Geometry check sheet. Reference: the model listing, model coordinates, mm. Face numbers are marked on the shaded views. A direction names the side the tool comes from. Round coordinates to 2 decimals unless told otherwise and drop trailing zeros. Loops run counter-clockwise (first coordinate to the right, second up) from the corner with the lowest first, then second, coordinate; pieces in that order, holes last.
```python
from build123d import *
from build123d.topology import SkipClean

# Parameters (mm, degrees)
ESQUISSE1_R        = 75
ESQUISSE1_R_2      = 2
BOSS_EXTRU_1_DEPTH = 10
ESQUISSE2_R        = 2
ESQUISSE2_W        = 21
ESQUISSE2_H        = 41
ESQUISSE2_H_2      = 6.85
BOSS_EXTRU_2_DEPTH = 2
BOSS_EXTRU_5_START = 2
ESQUISSE2_7_R      = 2
BOSS_EXTRU_5_DEPTH = 8


with BuildPart() as part:
    # Esquisse1 → Boss.-Extru.1 (new body)
    with BuildSketch(Plane(origin=(0, 0, 0), x_dir=(1, 0, 0), z_dir=(0, 1, 0))):
        with Locations(Location((0, 0, 0), (0, 0, 270))):
            Circle(ESQUISSE1_R)
        with Locations(Location((0, 65, 0), (0, 0, 270))):
            Circle(ESQUISSE1_R_2, mode=Mode.SUBTRACT)
        with Locations(Location((0, -65, 0), (0, 0, 270))):
            Circle(ESQUISSE1_R_2, mode=Mode.SUBTRACT)
    extrude(amount=BOSS_EXTRU_1_DEPTH)

    # Esquisse2 → Boss.-Extru.2 (add)
    # profile 1 of 3: a face of its own
    with BuildSketch(Plane.XY):
        with BuildLine():
            ThreePointArc((-25.073934757, 16.568086991), (-23.205708304, 20.950030541), (-23.576750129, 25.699138596))
            Line((-23.576750129, 25.699138596), (-28.491553882, 40.606845184))
            ThreePointArc((-28.491553882, 40.606845184), (0, 80), (28.491553882, 40.606845184))
            Line((28.491553882, 40.606845184), (23.576750129, 25.699138596))
            ThreePointArc((23.576750129, 25.699138596), (23.205708304, 20.950030541), (25.073934757, 16.568086991))
            Line((25.073934757, 16.568086991), (30, 10))
            Line((30, 10), (-30, 10))
            Line((-30, 10), (-25.073934757, 16.568086991))
        make_face()
        with Locations((4.751288604, 21.76470447)):
            Circle(ESQUISSE2_R, mode=Mode.SUBTRACT)
        with Locations((-5.248711396, 21.76470447)):
            Circle(ESQUISSE2_R, mode=Mode.SUBTRACT)
        with Locations((-5.248711396, 70.39470447)):
            Circle(ESQUISSE2_R, mode=Mode.SUBTRACT)
        with Locations((4.751288604, 70.39470447)):
            Circle(ESQUISSE2_R, mode=Mode.SUBTRACT)
        with Locations((-0.248711396, 46.01543183)):
            Rectangle(ESQUISSE2_W, ESQUISSE2_H, mode=Mode.SUBTRACT)
    # profile 2 of 3: a face of its own
    with BuildSketch(Plane.XY):
        with Locations((-0.248711396, 69.94043183)):
            Rectangle(ESQUISSE2_W, ESQUISSE2_H_2)
        with Locations((-5.248711396, 70.39470447)):
            Circle(ESQUISSE2_R, mode=Mode.SUBTRACT)
        with Locations((4.751288604, 70.39470447)):
            Circle(ESQUISSE2_R, mode=Mode.SUBTRACT)
    # profile 3 of 3: a face of its own
    with BuildSketch(Plane.XY):
        with BuildLine():
            Line((10.251288604, 73.36543183), (10.251288604, 78.194167517))
            ThreePointArc((10.251288604, 78.194167517), (-0.265506097, 79.998825086), (-10.748711396, 78.00830597))
            Line((-10.748711396, 78.00830597), (-10.748711396, 73.36543183))
            Line((-10.748711396, 73.36543183), (10.251288604, 73.36543183))
        make_face()
    extrude(amount=BOSS_EXTRU_2_DEPTH)

    # Esquisse2<7> → Boss.-Extru.5 (add)
    with SkipClean():  # the faces are left unmerged after this step: merging them gives an invalid solid
        with BuildSketch(Plane.XY.offset(BOSS_EXTRU_5_START)):
            with BuildLine():
                Line((23.576750129, 25.699138596), (28.491553882, 40.606845184))
                ThreePointArc((28.491553882, 40.606845184), (26.989880715, 63.097569965), (10.251288604, 78.194167517))
                Line((10.251288604, 78.194167517), (10.251288604, 73.36543183))
                Line((10.251288604, 73.36543183), (10.251288604, 66.51543183))
                Line((10.251288604, 66.51543183), (10.251288604, 25.51543183))
                Line((10.251288604, 25.51543183), (-10.748711396, 25.51543183))
                Line((-10.748711396, 25.51543183), (-10.748711396, 66.51543183))
                Line((-10.748711396, 66.51543183), (-10.748711396, 73.36543183))
                Line((-10.748711396, 73.36543183), (-10.748711396, 78.00830597))
                ThreePointArc((-10.748711396, 78.00830597), (-27.104739844, 62.858191085), (-28.491553882, 40.606845184))
                Line((-28.491553882, 40.606845184), (-23.576750129, 25.699138596))
                ThreePointArc((-23.576750129, 25.699138596), (-23.205708304, 20.950030541), (-25.073934757, 16.568086991))
                Line((-25.073934757, 16.568086991), (-30, 10))
                Line((-30, 10), (30, 10))
                Line((30, 10), (25.073934757, 16.568086991))
                ThreePointArc((25.073934757, 16.568086991), (23.205708304, 20.950030541), (23.576750129, 25.699138596))
            make_face()
            with Locations((-5.248711396, 21.76470447)):
                Circle(ESQUISSE2_7_R, mode=Mode.SUBTRACT)
            with Locations((4.751288604, 21.76470447)):
                Circle(ESQUISSE2_7_R, mode=Mode.SUBTRACT)
        extrude(amount=BOSS_EXTRU_5_DEPTH)


solid = part.part
```
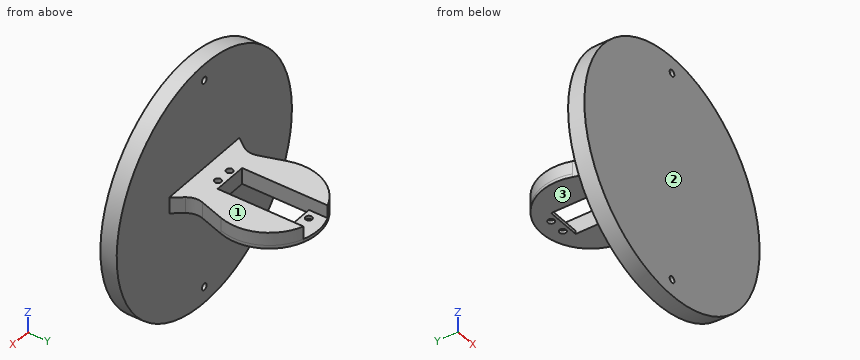
1) Sectioned sample at A-A, the plane y = 55. Record the cut outline in (x, z).
Report:
outline: (-29.58, 0) - (-10.75, 0) - (-10.75, 10) - (-29.58, 10) - close; (10.25, 0) - (29.58, 0) - (29.58, 10) - (10.25, 10) - close
2) Access from +Z, -Z, +X, -X, +Y, -Y to the whole of each face (thin tool, end or side, straight path). Record for the marked faces 1, 2 and 3.
Report:
face 1: +Z, +X, -X, +Y
face 2: +Z, -Z, +X, -X, -Y
face 3: -Z, +X, -X, +Y
3) Sectioned sample at B-B, the plane z = 65. Record the cut outline in (x, y), then the cut area to 3 significant figures.
Report:
outline: (-37.42, 0) - (-2, 0) - (-2, 10) - (-37.42, 10) - close; (2, 0) - (37.42, 0) - (37.42, 10) - (2, 10) - close
area: 708 mm2
4) Scan lines: line 1 along Z through (x, y) = (10, 71); line 2 along Y through (x, z) = (12, 56.5). Record each from-to range of solid material in increasing order.
Report:
line 1: z = 0 to 2
line 2: y = 0 to 10
5) Gauge pin test, flat ends, axial feed: pin 1 (2 mm diameter, centred on x = -2.5, z = -16, fed in from +Y); pin 2 (6 mm diameter, centred on y = 9, z = -48, fed in from -X); pin 3 (5 mm diameter, centred on x = 4.75, y = 21.76, fed in from +Z); pin 4 (6.5 mm diameter, centred on x = 0, z = 65, fed in from -Y). Record the tip position at first contact, or that the pin passes through.
Report:
pin 1: stops at y = 10
pin 2: stops at x = -60
pin 3: stops at z = 10
pin 4: stops at y = 0
6) Sectioned sample at D-D, the plane y = 46. Record the cut outline in (x, z), then the cut area to 3 significant figures.
Report:
outline: (-29.73, 0) - (-10.75, 0) - (-10.75, 10) - (-29.73, 10) - close; (10.25, 0) - (29.73, 0) - (29.73, 10) - (10.25, 10) - close
area: 385 mm2
7) Sectioned sample at C-C, the plane x = -45. Record the cut outline in (y, z).
Report:
outline: (0, -60) - (10, -60) - (10, 60) - (0, 60) - close
